from build123d import *

# Parameters (mm, degrees)
SKETCH2_W               = 88.9
SKETCH2_H               = 152.4
BOSS_EXTRUDE1_DEPTH     = 5.9944
SKETCH3_R               = 1.905
CUT_EXTRUDE1_DEPTH      = 1
CUT_EXTRUDE1_DEPTH_BACK = 6.9944
SKETCH4_R               = 2.7305
CUT_EXTRUDE2_DEPTH      = 1
CUT_EXTRUDE2_DEPTH_BACK = 6.9944


with BuildPart() as part:
    # Sketch2 → Boss-Extrude1 (new body)
    with BuildSketch(Plane(origin=(0, 0, 0), x_dir=(1, 0, 0), z_dir=(0, 1, 0))):
        with Locations((44.45, 76.2)):
            Rectangle(SKETCH2_W, SKETCH2_H)
    extrude(amount=BOSS_EXTRUDE1_DEPTH)

    # Sketch3 → Cut-Extrude1 (cut, two sides)
    with BuildSketch(Plane(origin=(0, 5.9944, 0), x_dir=(1, 0, 0), z_dir=(0, 1, 0))) as cut_extrude1_sk:
        with Locations((52.07, 147.193)):
            Circle(SKETCH3_R)
        with Locations((3.81, 139.7)):
            Circle(SKETCH3_R)
        with Locations((3.81, 64.5668)):
            Circle(SKETCH3_R)
        with Locations((52.07, 64.5668)):
            Circle(SKETCH3_R)
        with Locations((48.3362, 53.2638)):
            Circle(SKETCH3_R)
        with Locations((85.09, 53.2638)):
            Circle(SKETCH3_R)
        with Locations((48.3362, 16.51)):
            Circle(SKETCH3_R)
        with Locations((85.09, 16.51)):
            Circle(SKETCH3_R)
    extrude(amount=CUT_EXTRUDE1_DEPTH, mode=Mode.SUBTRACT)
    extrude(cut_extrude1_sk.sketch, amount=-CUT_EXTRUDE1_DEPTH_BACK, mode=Mode.SUBTRACT)

    # Sketch4 → Cut-Extrude2 (cut, two sides)
    with BuildSketch(Plane(origin=(0, 5.9944, 0), x_dir=(1, 0, 0), z_dir=(0, 1, 0))) as cut_extrude2_sk:
        with Locations((45.72, 109.871331367)):
            Circle(SKETCH4_R)
        with Locations((45.72, 33.671331367)):
            Circle(SKETCH4_R)
    extrude(amount=CUT_EXTRUDE2_DEPTH, mode=Mode.SUBTRACT)
    extrude(cut_extrude2_sk.sketch, amount=-CUT_EXTRUDE2_DEPTH_BACK, mode=Mode.SUBTRACT)


solid = part.part
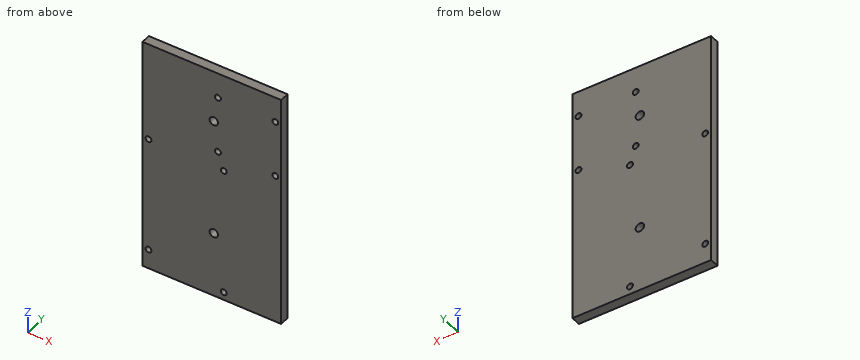
Geometry: final body of the model. Coordinates: model frame, mm. Round coordinates to 2 decimals unless told otherwise and drop trailing zeros. Loops run counter-clockwise (first coordinate to the right, second up) from the corner with the lowest first, then second, coordinate; pieces in that order, holes last. Notation, with made-up numbers: M -38.75,30 L 15.25,30 A29 ccw 15.25,52 Z; hole C -38,-17.5 d11. An arc over 180 degrees is marked long. One line per question, with ' | ' between items.
(1) Material intervals for line 1 along Z through (x, y) = (3.81, 3.2) (3 decimals); line 2 along Z through (x, y) = (85.09, 3.75) (3 decimals); line 3 along X through (y, z) = (3.6, -16.51) (3 decimals), sorted ascending. Write a range as from..to.
Check result:
line 1: z = -152.4..-141.605, -137.795..-66.472, -62.662..0 | line 2: z = -152.4..-55.169, -51.359..-18.415, -14.605..0 | line 3: x = 0..46.431, 50.241..83.185, 86.995..88.9
(2) Contact query for a flat-ended pin moving along its axis: P1, Ø3, axis at x = 85.09, z = -16.51, coming from the +Y side. Output: stop coordinate, or through.
Check result:
P1: passes through
(3) Cut plane C-C on z = -139.7. Return the cut outline in (x, y) (3 decimals).
Check result:
outline: M 0,0 L 1.905,0 L 1.905,5.994 L 0,5.994 Z; M 5.715,0 L 88.9,0 L 88.9,5.994 L 5.715,5.994 Z
(4) Cut plane B-B on x = 85.09. Return the cut outline in (y, z) (3 decimals), plus the area to 3 significant figures.
Check result:
outline: M 0,-152.4 L 5.994,-152.4 L 5.994,-55.169 L 0,-55.169 Z; M 0,-51.359 L 5.994,-51.359 L 5.994,-18.415 L 0,-18.415 Z; M 0,-14.605 L 5.994,-14.605 L 5.994,0 L 0,0 Z | area: 868 mm2
(5) Cut plane A-A on z = -16.51. Return the cut outline in (x, y) (3 decimals), plus the area to 3 significant figures.
Check result:
outline: M 0,0 L 46.431,0 L 46.431,5.994 L 0,5.994 Z; M 50.241,0 L 83.185,0 L 83.185,5.994 L 50.241,5.994 Z; M 86.995,0 L 88.9,0 L 88.9,5.994 L 86.995,5.994 Z | area: 487 mm2
